Autodesk Inventor part; units mm, degrees
ref_plane "YZ Plane" through (0, 0, 0) normal (1, 0, 0) x (0, 1, 0)
ref_plane "XZ Plane" through (0, 0, 0) normal (0, 1, 0) x (-1, 0, 0)
ref_plane "XY Plane" through (0, 0, 0) normal (0, 0, 1) x (1, 0, 0)
sketch "Sketch1" plane through (0, 0, 0) normal (1, 0, 0) x (0, 1, 0)
  line L0 (15, 143.75) -> (-15, 143.75)
  line L1 (-15, 143.75) -> (-15, -143.75)
  line L2 (-15, -143.75) -> (15, -143.75)
  line L3 (15, -143.75) -> (15, 143.75)
  point P0 (0, 0)
  dimension "d0" = 287.5
  dimension "d1" = 143.75
  dimension "d2" = 30
  dimension "d3" = 15
extrude "Extrusion1" add sketch "Sketch1" along normal blind 30
fillet "Fillet1" radius 2 4 edges at (0, 15, 0) (0, -15, 0) (30, -15, 0) (30, 15, 0)
sketch "Sketch2" plane through (0, -13, -143.75) normal (0, 0, -1) x (-1, 0, 0)
  line L0 (-27.5, 25.5) -> (-2.5, 25.5)
  line L1 (-2.5, 25.5) -> (-2.5, 0.5)
  line L2 (-2.5, 0.5) -> (-27.5, 0.5)
  line L3 (-27.5, 0.5) -> (-27.5, 25.5)
  line L4 (-2, 28) -> (-28, 28)
  line L5 (-2, -2) -> (-28, -2)
  line L6 (0, 0) -> (0, 26)
  line L7 (-30, 0) -> (-30, 26)
  point P0 (0, 13)
  dimension "d7" = 2.5
  dimension "d8" = 2.5
  dimension "d9" = 2.5
  dimension "d10" = 2.5
extrude "Extrusion2" cut sketch "Sketch2" against normal blind 300
fillet "Fillet2" radius 2 4 edges at (27.5, -12.5, 0) (27.5, 12.5, 0) (2.5, 12.5, 0) (2.5, -12.5, 0)
equation "\"d0\" = 0.5 * wheelchair_deployed_width - secure_arm_hold_thickness"
equation "\"d2\" = secure_arm_hold_thickness"
equation "\"d4\" = secure_arm_hold_thickness"
equation "\"hoop_angle_z\" = 45deg"
equation "\"hoop_bearing_length\" = 5deg"
equation "\"hoop_cable_diam\" = 5"
equation "\"hoop_cable_pulley_diam\" = 22"
equation "\"hoop_thickness_large\" = 4"
equation "\"hoop_thickness_medium\" = 3.2"
equation "\"hoop_thickness_small\" = 2"
equation "\"hoop_width_large\" = 51"
equation "\"hoop_width_medium\" = 33.7"
equation "\"hoop_width_small\" = 25.4"
equation "\"rack_tooth_addendum\" = 5"
equation "\"rack_tooth_dedendum\" = 5"
equation "\"rack_tooth_thickness\" = 5"
equation "\"secure_arm_angle\" = 35deg"
equation "\"secure_arm_hold_thickness\" = 30"
equation "\"secure_arm_radii\" = 9"
equation "\"support_baseClamp_platformLengthBuffer\" = 35"
equation "\"support_baseClamp_platformThickness\" = 15"
equation "\"support_baseClamp_platformWidthBuffer\" = 0"
equation "\"support_baseClamp_sleeveHoleDiameter\" = 12"
equation "\"support_baseClamp_sleeveSweepTerminationAngle\" = 55deg"
equation "\"support_baseClamp_thickness\" = 8"
equation "\"support_frame_endHoleBuffer\" = 45"
equation "\"support_frame_squareBarFillet\" = 2"
equation "\"support_frame_squareBarThickness\" = 5"
equation "\"hoop_tabs_thickness\" = 6"
equation "\"hoop_tabs_hole\" = 12"
equation "\"wheelchair_deployed_width\" = 635"
equation "\"wheelchair_deployed_height\" = 914"
equation "\"wheelchair_deployed_length\" = 1067"
equation "\"sm_varx_pinPlate_thickness\" = 5"
equation "\"sm_varx_member_tolerance\" = 0"
equation "\"sm_varx_pinPlate_holeDiameter\" = 5"
equation "\"sm_varx_squareBarThickness\" = 2.5"
equation "\"hoop_bushing23_radialInterference\" = 0"
equation "\"hoop_bushing12_radialInterference\" = 0"
equation "\"hoop_bushing12_od\" = -2 * hoop_thickness_large + hoop_width_large + hoop_bushing12_radialInterference"
equation "\"hoop_bushing23_od\" = -2 * hoop_thickness_medium + hoop_width_medium + hoop_bushing23_radialInterference"
equation "\"wheelchatir_pos_deploy_angle_0\" = 65deg"
equation "\"wheelchatir_pos_store_angle_0\" = 90deg"
equation "\"wheelchatir_pos_deploy_angle_1\" = 20deg"
equation "\"wheelchatir_pos_store_angle_1\" = 20deg"
equation "\"hoop_bushing12_thickness\" = -hoop_width_medium + hoop_bushing12_od - 2 * hoop_bushing12_radialInterference"
equation "\"hoop_bushing23_thickness\" = -hoop_width_small + hoop_bushing23_od - 2 * hoop_bushing23_radialInterference"
properties part number "secure_width_bar"
Geometry: final body of the model. Coordinates: model frame, mm. A direction names the side the tool comes from. Round coordinates to 2 decimals unless told otherwise and drop trailing zeros. Order: outer loops, then holes, each group sorted by start corner. A loop starts at its lowest first (then second) coordinate and runs counter-clockwise, first axis right, second up. Notation, with made-up numbers: (25, -3.5) -> (57, -3.5) arc R21 ccw to (57, 19.5) -> close; hole circle Ø6 at (-2, -24). An arc over 180 degrees is marked (long way). Put each result on its own line as item: value. Start each with the question number.
Q1. Section A-A on y = 3.5. Return the cut outline in (x, z).
Q2. Section C-C on z = -77.5. Return the cut outline in (x, y), and give its area (3 significant figures).
Q3. Pull-direction query (Y, two-part tool) for faces 3 (the flat face through (0, 0, 2)), 4 (the flat face through (15, -15, 2)), 5 (the flat face through (15, -12.5, -2)); classes: +Y half, -Y half, draft (parallel to the pull), parting line (faces both ways), or undercut.
Q4. Line query: probe 1 along X at (y, z) = (-10.25, -103); probe 2 along Y at (x, z) = (20.25, -18); probe 3 along Y at (x, z) = (26.5, 65.5). Output: solid intervals per line, ascending.
Q5. Section B-B on x = 12. Return the cut outline in (y, z).
Q6. First-contact query: pin 1 (4 mm diameter, centred on x = 11, y = -11.5, fed in from +Z). Flat tip, straight axial feed; report the tip coordinate or a pass-through.
Q7. Reachability of faces 1 (the flat face through (27.5, 0, -2)), 2 (the flat face through (15, -14, -143.75)) from +Z, -Z, +X, -X, +Y, -Y: full face, straight path, thin tool, end or side. Return the list, or none.
Ans:
1. outline: (0, -143.75) -> (2.5, -143.75) -> (2.5, 143.75) -> (0, 143.75) -> close; (27.5, -143.75) -> (30, -143.75) -> (30, 143.75) -> (27.5, 143.75) -> close
2. outline: (0, -13) arc R2 ccw to (2, -15) -> (28, -15) arc R2 ccw to (30, -13) -> (30, 13) arc R2 ccw to (28, 15) -> (2, 15) arc R2 ccw to (0, 13) -> close; hole (2.5, -10.5) arc R2 ccw to (4.5, -12.5) -> (25.5, -12.5) arc R2 ccw to (27.5, -10.5) -> (27.5, 10.5) arc R2 ccw to (25.5, 12.5) -> (4.5, 12.5) arc R2 ccw to (2.5, 10.5) -> close
2. area: 275 mm2
3. face 3: draft
3. face 4: -Y half
3. face 5: undercut
4. probe 1: x = 0 to 2.5, 27.5 to 30
4. probe 2: y = -15 to -12.5, 12.5 to 15
4. probe 3: y = -15 to -12.23, 12.23 to 15
5. outline: (-15, -143.75) -> (-12.5, -143.75) -> (-12.5, 143.75) -> (-15, 143.75) -> close; (12.5, -143.75) -> (15, -143.75) -> (15, 143.75) -> (12.5, 143.75) -> close
6. pin 1: stops at z = 143.75
7. face 1: +Z, -Z
7. face 2: -Z, +X, -X, +Y, -Y
